Here's the drawing with two shaded views (mm, measured from the low corner). I have some questions. A direction names the side the tool comes from. Round coordinates to 2 decimals unless told otherwise and drop trailing zeros. Loops run counter-clockwise (first coordinate to the right, second up) from the corner with the lowest first, then second, coordinate; pieces in that order, holes last. Notation, with made-up numbers: M 83.5,35 L 129.5,35 A21 ccw 129.5,51 Z; hole C 39,52 d6. An arc over 180 degrees is marked long. One line per item, written item: value. Start each with the question number.
Q1. Imagine slicing it at C-C (y = 14). Please give me the cut outline in (x, z).
Q2. Which directions (+Z, -Z, +X, -X, +Y, -Y) give clear straight access to the entire face, cutting with the end or side of a thin tool? Please do the marked faces 5, 6, 7 and 8.
Q3. Imagine slicing it at B-B (x = 38). Please give me the cut outline in (y, z), then the cut area to 3 significant figures.
Q4. Imagine slicing it at A-A (x = 52.6). Please give me the cut outline in (y, z), then the cut area to 3 significant figures.
Q5. I'm going to push flat-ended pins straight in: pin 1 Ø1.5 at (y, z) = (14.5, 23.5) entering from +X; pin 2 Ø6 at (x, y) = (19, 8) entering from -Z; pin 3 Ø4 at (x, y) = (52.6, 3) entering from -Z. Where does each tip first touch, or does it pass through?
Q6. Please list where these lines run through material, in increasing order: line 1 along Z through (x, y) = (48.5, 16.5); line 2 along X through (y, z) = (7, 39); line 3 along Z through (x, y) = (42.5, 15).
Q7. Thinking about a two-plate mould opening in Y: for the marked faces 1, 2, 3 and 4, which applies, released by +Y, released by -Y, zero draft, split by the parting line, or undercut?
Q8. Imagine slicing it at D-D (z = 21). Please give me the cut outline in (x, y), then the cut area to 3 significant figures.
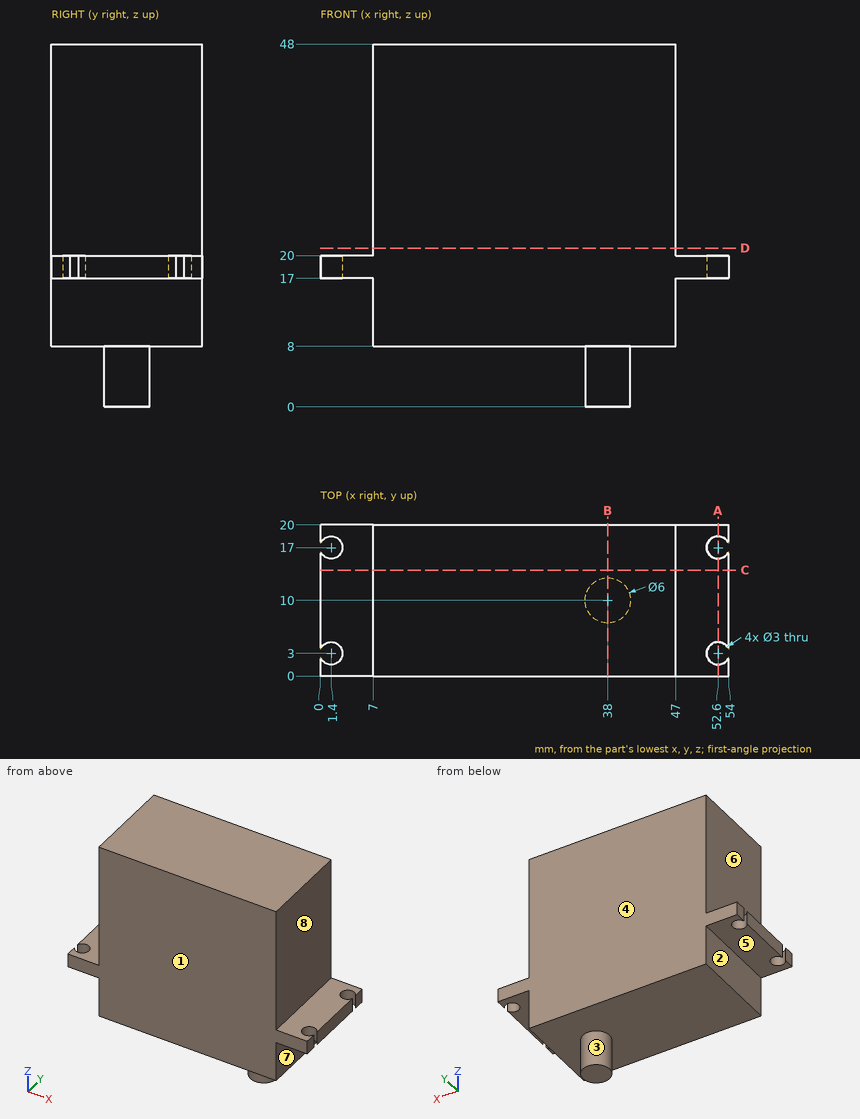
Report:
1. outline: M 0,17 L 7,17 L 7,8 L 47,8 L 47,17 L 54,17 L 54,20 L 47,20 L 47,48 L 7,48 L 7,20 L 0,20 Z
2. face 5: -Z, -X, +Y, -Y
2. face 6: +Z, -X, +Y, -Y
2. face 7: -Z, +X, +Y, -Y
2. face 8: +Z, +X, +Y, -Y
3. outline: M 0,8 L 7,8 L 7,0 L 13,0 L 13,8 L 20,8 L 20,48 L 0,48 Z
3. area: 848 mm²
4. outline: M 0,17 L 1.5,17 L 1.5,20 L 0,20 Z; M 4.5,17 L 15.5,17 L 15.5,20 L 4.5,20 Z; M 18.5,17 L 20,17 L 20,20 L 18.5,20 Z
4. area: 42.0 mm²
5. pin 1: stops at x = 47
5. pin 2: stops at z = 8
5. pin 3: stops at z = 17
6. line 1: z = 17 to 20
6. line 2: x = 7 to 47
6. line 3: z = 8 to 48
7. face 1: released by -Y
7. face 2: zero draft
7. face 3: split by the parting line
7. face 4: released by +Y
8. outline: M 7,0 L 47,0 L 47,20 L 7,20 Z
8. area: 800 mm²
